Source: CAD feature listing. Evaluate the final solid. Frame: model axes, mm. Face numbers are marked on the shaded views. Round coordinates to 2 decimals unless told otherwise and drop trailing zeros. Loops run counter-clockwise (first coordinate to the right, second up) from the corner with the lowest first, then second, coordinate; pieces in that order, holes last. Notation, with made-up numbers: (24, -14) - (83, -14) arc R19 cw to (83, 6) - close; hole circle Ø1 at (-22.75, 37.25). An arc over 180 degrees is marked (long way). Write item = value, one per line. Start each with the question number.
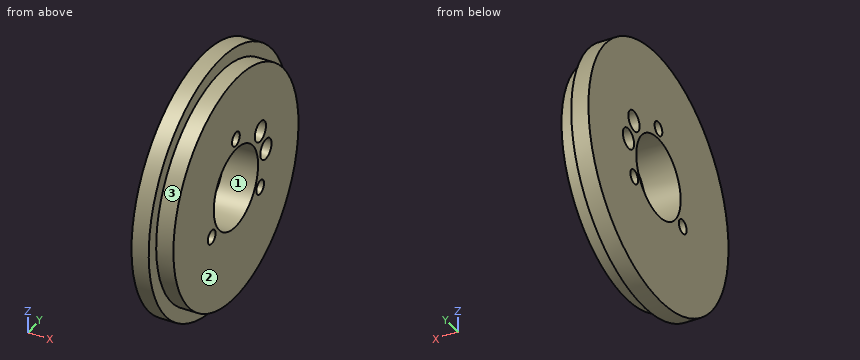
from build123d import *

# Parameters (mm, degrees)
AXIAL_HOLES_DEPTH      = 150.832206151
AXIAL_HOLES_DEPTH_BACK = 150.832206151
SKETCH2_R              = 2.4
SKETCH2_R_2            = 1.65


with BuildPart() as part:
    # Axial profile (mm) → Full revolution (revolve)
    with BuildSketch(Plane.XY, mode=Mode.PRIVATE) as full_revolution_sk:
        Polygon((135.7, 9.5), (143.7, 9.5), (143.7, 26.8), (139.7, 26.8), (139.7, 30), (135.7, 30), align=None)
    revolve(full_revolution_sk.sketch.rotate(Axis((-110, 0, 0), (1, 0, 0)), 90), axis=Axis((-110, 0, 0), (1, 0, 0)))

    # Sketch2 → Axial holes (cut, two sides: drawn at the far end of the back side and taken through both)
    with BuildSketch(Plane(origin=(0, 0, 0), x_dir=(0, 0, -1), z_dir=(1, 0, 0)).offset(-AXIAL_HOLES_DEPTH_BACK)):
        with Locations((-1.977382665, 12.848733704)):
            Circle(SKETCH2_R)
        with Locations((-7.687206041, 10.483647423)):
            Circle(SKETCH2_R)
        with Locations((-12, 0)):
            Circle(SKETCH2_R_2)
        with Locations((6, -10.392304845)):
            Circle(SKETCH2_R_2)
        with Locations((6, 10.392304845)):
            Circle(SKETCH2_R_2)
    extrude(amount=AXIAL_HOLES_DEPTH + AXIAL_HOLES_DEPTH_BACK, mode=Mode.SUBTRACT)


solid = part.part
(1) Pin query (flat end, axial travel): P1, Ø1, axis at x = 142, y = 15, coming from the +Z side; P2, Ø11.5, axis at y = 0, z = 0, coming from the +X side; P3, Ø1.5, axis at x = 141, y = 23, coming from the +Z side; P4, Ø3, axis at x = 138.5, z = 23.5, coming from the +Y side. Return the tip coordinate at first contact, or that it passes through.
(2) Cut plane C-C (x = 136.5). Output: boundary loops of the cut face in (y, z).
(3) Material intervals for line 1 along Y through (x, z) = (141.5, -6); line 2 along Y through (x, z) = (143, 3); line 3 along Z through (x, y) = (138.25, 11), sorted ascending. Write a range as from..to.
(4) Mould query, pull axis Y, two halves, no side actions, for the marked faces 1, 2 and 3. Classes: +Y half, -Y half, draft (parallel to the pull), parting line (faces both ways), or undercut.
(5) Cut plane D-D (z = -19). Output: boundary loops of the cut face in (x, y), and give its area (3 significant figures).
(6) Cut plane A-A (y = 0). Output: boundary loops of the cut face in (x, z).
(7) Cut plane B-B (z = -3). Output: boundary loops of the cut face in (x, y).
Solution:
q1.P1 = 22.54
q1.P2 = through
q1.P3 = 14.94
q1.P4 = 20.4
q2.outline = circle Ø60 at (0, 0); hole circle Ø3.3 at (-10.39, -6); hole circle Ø19 at (0, 0); hole circle Ø3.3 at (0, 12); hole circle Ø4.8 at (10.48, 7.69); hole circle Ø3.3 at (10.39, -6); hole circle Ø4.8 at (12.85, 1.98)
q3.line_1 = -26.12..-12.04, -8.74..-7.37, 7.37..8.74, 12.04..26.12
q3.line_2 = -26.63..-9.01, 9.01..10.68, 15.02..26.63
q3.line_3 = -27.91..-7.53, -4.47..0.45, 3.51..5.34, 10.03..27.91
q4.face_1 = undercut
q4.face_2 = draft
q4.face_3 = parting line
q5.outline = (135.7, -23.22) - (139.7, -23.22) - (139.7, -18.9) - (143.7, -18.9) - (143.7, 18.9) - (139.7, 18.9) - (139.7, 23.22) - (135.7, 23.22) - close
q5.area = 337 mm^2
q6.outline = (135.7, -30) - (139.7, -30) - (139.7, -26.8) - (143.7, -26.8) - (143.7, -9.5) - (135.7, -9.5) - close; (135.7, 9.5) - (143.7, 9.5) - (143.7, 10.35) - (135.7, 10.35) - close; (135.7, 13.65) - (143.7, 13.65) - (143.7, 26.8) - (139.7, 26.8) - (139.7, 30) - (135.7, 30) - close
q7.outline = (135.7, -29.85) - (139.7, -29.85) - (139.7, -26.63) - (143.7, -26.63) - (143.7, -9.01) - (135.7, -9.01) - close; (135.7, 9.01) - (143.7, 9.01) - (143.7, 26.63) - (139.7, 26.63) - (139.7, 29.85) - (135.7, 29.85) - close
